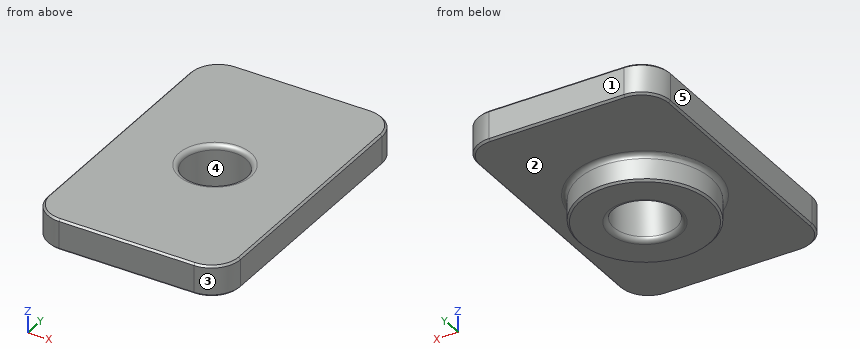
Autodesk Inventor part; units mm, degrees
ref_plane "YZ Plane" through (0, 0, 0) normal (1, 0, 0) x (0, 1, 0)
ref_plane "XZ Plane" through (0, 0, 0) normal (0, 1, 0) x (-1, 0, 0)
ref_plane "XY Plane" through (0, 0, 0) normal (0, 0, 1) x (1, 0, 0)
sketch "Sketch1" plane through (0, 0, 0) normal (0, 0, 1) x (1, 0, 0)
  line L0 (5, -7.5) -> (-5, -7.5)
  line L1 (-5, -7.5) -> (-5, 7.5)
  line L2 (-5, 7.5) -> (5, 7.5)
  line L3 (5, 7.5) -> (5, -7.5)
  line L4 (5, -7.5) -> (-5, 7.5) construction
  line L5 (-5, -7.5) -> (5, 7.5) construction
  point P0 (0, 0)
  dimension "d0" = 10
  dimension "d1" = 15
extrude "Extrusion1" add sketch "Sketch1" against normal blind 1.6
sketch "Sketch2" plane through (0, 0, -1.6) normal (0, 0, -1) x (-1, 0, 0)
  circle A0 centre (0, 0) radius 3.45
  dimension "d4" = 6.9
extrude "Extrusion2" add sketch "Sketch2" along normal blind 1.4
fillet "Fillet1" radius 0.25 1 edges at (3.45, 0, -1.6)
fillet "Fillet2" radius 1.5 4 edges at (5, 7.5, -0.8) (-5, 7.5, -0.8) (-5, -7.5, -0.8) (5, -7.5, -0.8)
sketch "Sketch3" plane through (0, 0, -3) normal (0, 0, -1) x (-1, 0, 0)
  circle A0 centre (0, 0) radius 3.45
hole "Hole1" at (0, 0, -3) direction (0, 0, 1) diameter 3.242 end through all
fillet "Fillet3" radius 0.25 2 edges at (0, -1.621, 0) (0, -1.621, -3)
chamfer "Chamfer1" distance 0.1 angle 45 1 edges at (3.45, 0, -3)
chamfer "Chamfer2" distance 0.1 angle 45 16 edges at (4.5607, 7.0607, 0) (5, 0, 0) (4.5607, -7.0607, 0) (0, -7.5, 0) (-4.5607, -7.0607, 0) (-5, 0, 0) (-4.5607, 7.0607, 0) (0, 7.5, 0) (4.5607, 7.0607, -1.6) (0, 7.5, -1.6) (-4.5607, 7.0607, -1.6) (-5, 0, -1.6) (-4.5607, -7.0607, -1.6) (0, -7.5, -1.6) (4.5607, -7.0607, -1.6) (5, 0, -1.6)
properties part number "M4 T SLOT NUT"
The listing builds one solid part. Answer for the finished solid, in the listing's coordinates (mm). Face numbers are marked on the shaded views. A direction names the side the tool comes from. Give positions to 0.01 mm unless a question says otherwise; leave off trailing zeros. Order: outer loops, then holes, each group sorted by start corner. A loop starts at its lowest first (then second) coordinate and runs counter-clockwise, first axis right, second up. Notation, with made-up numbers: (59, 67) - (75, 67) arc R24 cw to (75, 94) - close; hole circle Ø11 at (39, -33.5). An arc over 180 degrees is marked (long way). Use one line per item in the form item = value.
1) For the marked faces 1 and 2, determine the directions among +Z, -Z, +X, -X, +Y, -Y from which every point of the face is accessible in a straight line to the end or side of a thin tool.
Verdict:
face_1 = +Z, -Z, +X, -X, +Y
face_2 = -Z
2) Each of these flat-tipped pins is pushed along its axis until it touches: pin 1 (3 mm diameter, centred on x = 0, y = 0, fed in from +Z); pin 2 (1.5 mm diameter, centred on x = -2.5, y = 0.5, fed in from +Z). Where does it stop, or does it pass through?
Verdict:
pin_1 = through
pin_2 = 0
3) Find section A-A on x = 0. Determine the outline of the cut face in (y, z).
Verdict:
outline = (-7.5, -1.5) - (-7.4, -1.6) - (-3.7, -1.6) arc R0.25 cw to (-3.45, -1.85) - (-3.45, -2.9) - (-3.35, -3) - (-1.87, -3) arc R0.25 ccw to (-1.62, -2.75) - (-1.62, -0.25) arc R0.25 ccw to (-1.87, 0) - (-7.4, 0) - (-7.5, -0.1) - close; (1.62, -2.75) arc R0.25 ccw to (1.87, -3) - (3.35, -3) - (3.45, -2.9) - (3.45, -1.85) arc R0.25 cw to (3.7, -1.6) - (7.4, -1.6) - (7.5, -1.5) - (7.5, -0.1) - (7.4, 0) - (1.87, 0) arc R0.25 ccw to (1.62, -0.25) - close
4) Find section D-D on y = 5. Determine the outline of the cut face in (x, z).
Verdict:
outline = (-5, -1.5) - (-4.9, -1.6) - (4.9, -1.6) - (5, -1.5) - (5, -0.1) - (4.9, 0) - (-4.9, 0) - (-5, -0.1) - close
5) Find section C-C on z = -0.55. Determine the outline of the cut face in (x, y), and give its area (3 significant figures).
Verdict:
outline = (-5, -6) arc R1.5 ccw to (-3.5, -7.5) - (3.5, -7.5) arc R1.5 ccw to (5, -6) - (5, 6) arc R1.5 ccw to (3.5, 7.5) - (-3.5, 7.5) arc R1.5 ccw to (-5, 6) - close; hole circle Ø3.24 at (0, 0)
area = 140 mm^2
6) The mould has two halves that part along X. Classify the marked faces 3, 4 and 5: released by +X, released by -X, zero draft, split by the parting line, or undercut.
Verdict:
face_3 = released by +X
face_4 = undercut
face_5 = released by -X
7) Find section B-B on y = 0. Determine the outline of the cut face in (x, z).
Verdict:
outline = (-5, -1.5) - (-4.9, -1.6) - (-3.7, -1.6) arc R0.25 cw to (-3.45, -1.85) - (-3.45, -2.9) - (-3.35, -3) - (-1.87, -3) arc R0.25 ccw to (-1.62, -2.75) - (-1.62, -0.25) arc R0.25 ccw to (-1.87, 0) - (-4.9, 0) - (-5, -0.1) - close; (1.62, -2.75) arc R0.25 ccw to (1.87, -3) - (3.35, -3) - (3.45, -2.9) - (3.45, -1.85) arc R0.25 cw to (3.7, -1.6) - (4.9, -1.6) - (5, -1.5) - (5, -0.1) - (4.9, 0) - (1.87, 0) arc R0.25 ccw to (1.62, -0.25) - close
8) Consider probe 1 along X at (y, z) = (0, -0.95); probe 2 along Y at (x, z) = (0, -2.2); probe 3 along Z at (x, y) = (-0.5, 5.5). Determine where each line is inside the solid, lowest interval first. Write a range as [from, to].
Verdict:
probe_1 = [-5, -1.62], [1.62, 5]
probe_2 = [-3.45, -1.62], [1.62, 3.45]
probe_3 = [-1.6, 0]
